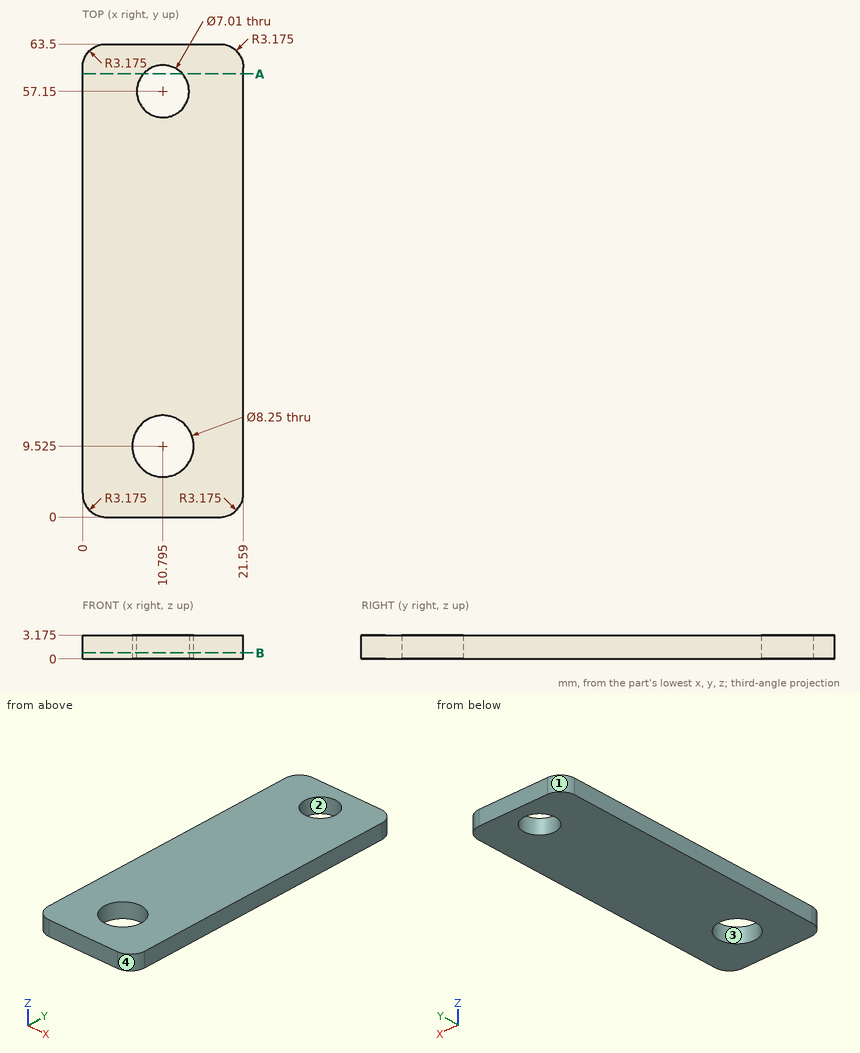
Answer from the drawing. Dimensions are ordinates in mm from the lowest x, y and z of the part. Round coordinates to 2 decimals unless told otherwise and drop trailing zeros. Write each loop counter-clockwise with the first axis right and the second up, starting at its lowest first coordinate (ties: lowest second). Pieces come first, ordered by that corner, then holes. Notation, with made-up numbers: (33.5, 81.25) -> (46.5, 81.25) arc R28 cw to (46.5, 100.25) -> close; hole circle Ø1 at (67.5, 4). An arc over 180 degrees is marked (long way). Answer in a Markdown table with one row per item. Add a question column.
1) Determine the mould class of the marked faces 1, 2, 3 and 4 for opening direction X: pulls with the +X half, pulls with the -X half, needs draft (parallel to the pull), parting line crosses it, or undercut.
2) Find section A-A, the plane y = 59.5. Determine the outline of the cut face in (x, z) (1 decimal).
3) Given P1, Ø10.5, axis at x = 10.795, y = 9.525, coming from the +Z side (3 decimals), flat-ended and moving along its own axis, determine where the tip first touches the part or whether it passes through.
4) Consider line 1 (Y direction, x = 13.25, z = 1.25); line 2 (Y direction, x = 9.75, z = 1.75) (1 decimal); line 3 (Y direction, x = 7, z = 2.1) (1 decimal). Determine where each line is inside the solid, lowest interval first.
5) Find section B-B, the plane z = 0.8. State how many separate pieces and enclosed holes the cut face has, and give its area (3 significant figures).
Findings below:
| question | item | result |
|---|---|---|
| 1 | face 1 | pulls with the -X half |
| 1 | face 2 | undercut |
| 1 | face 3 | undercut |
| 1 | face 4 | pulls with the +X half |
| 2 | outline | (0, 0) -> (8.2, 0) -> (8.2, 3.2) -> (0, 3.2) -> close; (13.4, 0) -> (21.6, 0) -> (21.6, 3.2) -> (13.4, 3.2) -> close |
| 3 | P1 | z = 3.175 |
| 4 | line 1 | 0 to 6.21, 12.84 to 54.65, 59.65 to 63.5 |
| 4 | line 2 | 0 to 5.5, 13.5 to 53.8, 60.5 to 63.5 |
| 4 | line 3 | 0 to 7.9, 11.1 to 63.5 |
| 5 | separate pieces | 1 |
| 5 | enclosed holes | 2 |
| 5 | area | 1,270 mm² |
